The figure shows three views and two pictorial views of one solid part (mm, origin at its lowest corner). Answer the questions. Coordinates: 2 decimals unless noted, no trailing zeros. Order: outer loops, then holes, each group sorted by start corner. A loop starts at its lowest first (then second) coordinate and runs counter-clockwise, first axis right, second up. Notation, with made-up numbers: (-33.75, -12.75) -> (-19.75, -12.75) arc R13 cw to (-19.75, -5.75) -> close; hole circle Ø6 at (2.25, 63). An arc over 180 degrees is marked (long way). Use one line per item in the form item = value.
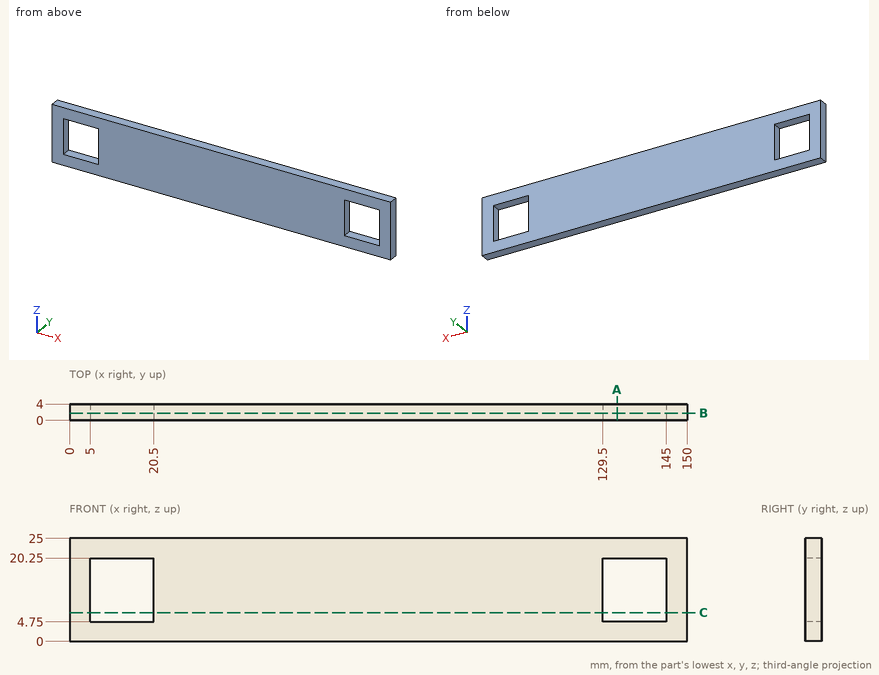
(1) Section C-C on z = 7 is taken. Write down the section's boundary in (x, y).
Data:
outline = (0, 0) -> (5, 0) -> (5, 4) -> (0, 4) -> close; (20.5, 0) -> (129.5, 0) -> (129.5, 4) -> (20.5, 4) -> close; (145, 0) -> (150, 0) -> (150, 4) -> (145, 4) -> close
(2) Section A-A on x = 133 is taken. Write down the section's boundary in (y, z), plus the area to 3 significant figures.
Data:
outline = (0, 0) -> (4, 0) -> (4, 4.75) -> (0, 4.75) -> close; (0, 20.25) -> (4, 20.25) -> (4, 25) -> (0, 25) -> close
area = 38.0 mm²
(3) This flat-tipped pin is pushed along its axis until it touches: P1, Ø6, axis at x = 94, z = 14, coming from the -Y side. Where does it stop, or does it pass through?
Data:
P1 = 0
(4) Section B-B on y = 1.8 is taken. Write down the section's boundary in (x, z), plus the area to 3 significant figures.
Data:
outline = (0, 0) -> (150, 0) -> (150, 25) -> (0, 25) -> close; hole (5, 4.75) -> (20.5, 4.75) -> (20.5, 20.25) -> (5, 20.25) -> close; hole (129.5, 4.75) -> (145, 4.75) -> (145, 20.25) -> (129.5, 20.25) -> close
area = 3,270 mm²
(5) Straight lines are drawn through the part: line 1 along X through (y, z) = (3.4, 9.5); line 2 along Z through (x, y) = (20, 0.6). For each, find the intervals that lie inside material, in ascending order.
Data:
line_1 = 0 to 5, 20.5 to 129.5, 145 to 150
line_2 = 0 to 4.75, 20.25 to 25
